Here's how the part is built. I have some questions about the finished solid (model axes, mm). Coordinates: 2 decimals unless noted, no trailing zeros. Write each loop counter-clockwise with the first axis right and the second up, starting at its lowest first coordinate (ties: lowest second). Pieces come first, ordered by that corner, then holes.
Item 1: If I drill on line 1 (X direction, y = 1, z = 0); line 2 (Z direction, x = -1.05, y = 0.5); line 3 (Y direction, x = 1.5, z = 1), over which ranges is the centre line in solid material (lowest first)?
Item 2: If we section it at D-D (z = 0): Please give me the cut outline in (x, y), then the cut area to 3 significant figures.
Item 3: If we section it at B-B (z = -1): Please give me the cut outline in (x, y).
Item 4: If we section it at A-A (x = 0): Please give me the cut outline in (y, z).
Item 5: If we section it at C-C (z = -3): Please give me the cut outline in (x, y).
Item 6: I'm going to push flat-ended pins straight in: pin 1 Ø4 at (y, z) = (6, -2) entering from -X; pin 2 Ø0.6 at (x, y) = (1, -2) entering from +Z; pin 3 Ø0.6 at (x, z) = (1, -2) entering from +Y. Where does each tip first touch, or does it pass through?
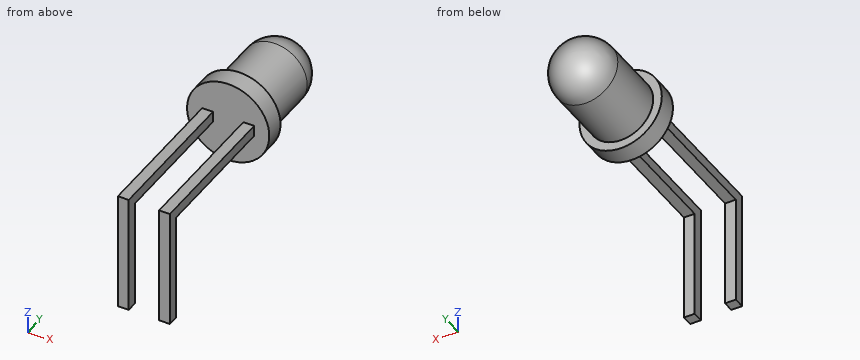
from build123d import *

# Parameters (mm, degrees)
SKICA2_W                = 0.5
SKICA2_H                = 6.8
P_IDAT_VYSUNUT_M1_DEPTH = 0.25
SKICA3_W                = 0.5
SKICA3_H                = 0.504797781
P_IDAT_VYSUNUT_M2_DEPTH = 5


with BuildPart() as part:
    # Skica1 → Rotovat1 (revolve)
    with BuildSketch(Plane.XY):
        with BuildLine():
            Line((-1.5, 6.066522781), (-1.5, 3.216522781))
            Line((-1.5, 3.216522781), (-1.9, 3.216522781))
            Line((-1.9, 3.216522781), (-1.9, 2.316522781))
            Line((-1.9, 2.316522781), (0, 2.316522781))
            Line((0, 2.316522781), (0, 7.566522781))
            ThreePointArc((0, 7.566522781), (-1.060660172, 7.127182953), (-1.5, 6.066522781))
        make_face()
    revolve(axis=Axis((0, 7.566522781, 0), (0, -1, 0)))

    # Skica2 → Přidat vysunutím1 (add, symmetric)
    with BuildSketch(Plane.XY):
        with Locations((0.95, -1.083477219)):
            Rectangle(SKICA2_W, SKICA2_H)
        with Locations((-0.95, -1.083477219)):
            Rectangle(SKICA2_W, SKICA2_H)
    extrude(amount=P_IDAT_VYSUNUT_M1_DEPTH, both=True)

    # Skica3 → Přidat vysunutím2 (add)
    with BuildSketch(Plane(origin=(0, 0, -0.25), x_dir=(-1, 0, 0), z_dir=(0, 0, -1))):
        with Locations((0.95, -4.231078329)):
            Rectangle(SKICA3_W, SKICA3_H)
        with Locations((-0.95, -4.231078329)):
            Rectangle(SKICA3_W, SKICA3_H)
    extrude(amount=P_IDAT_VYSUNUT_M2_DEPTH)


solid = part.part
Answer list:
1. line 1: x = -1.2 to -0.7, 0.7 to 1.2
1. line 2: z = -0.25 to 0.25
1. line 3: y = 2.32 to 3.22
2. outline: (-1.9, 2.32) - (-1.2, 2.32) - (-1.2, -4.48) - (-0.7, -4.48) - (-0.7, 2.32) - (0.7, 2.32) - (0.7, -4.48) - (1.2, -4.48) - (1.2, 2.32) - (1.9, 2.32) - (1.9, 3.22) - (1.5, 3.22) - (1.5, 6.07) arc R1.5 ccw to (-1.5, 6.07) - (-1.5, 3.22) - (-1.9, 3.22) - close
2. area: 22.3 mm2
3. outline: (-1.62, 2.32) - (1.62, 2.32) - (1.62, 3.22) - (1.12, 3.22) - (1.12, 6.07) arc R1.12 ccw to (-1.12, 6.07) - (-1.12, 3.22) - (-1.62, 3.22) - close; (-1.2, -4.48) - (-0.7, -4.48) - (-0.7, -3.98) - (-1.2, -3.98) - close; (0.7, -4.48) - (1.2, -4.48) - (1.2, -3.98) - (0.7, -3.98) - close
4. outline: (2.32, -1.9) - (3.22, -1.9) - (3.22, -1.5) - (6.07, -1.5) arc R1.5 ccw to (6.07, 1.5) - (3.22, 1.5) - (3.22, 1.9) - (2.32, 1.9) - close
5. outline: (-1.2, -4.48) - (-0.7, -4.48) - (-0.7, -3.98) - (-1.2, -3.98) - close; (0.7, -4.48) - (1.2, -4.48) - (1.2, -3.98) - (0.7, -3.98) - close
6. pin 1: stops at x = -1.5
6. pin 2: stops at z = 0.25
6. pin 3: stops at y = -3.98
